Read the model definition and answer for the solid it produces. Units are mm, in the model's axes. Give positions to 0.01 mm unless a question says otherwise; leave off trailing zeros. Loops run counter-clockwise (first coordinate to the right, second up) from the corner with the lowest first, then second, coordinate; pieces in that order, holes last.
(1) Find section C-C, the plane x = -19. Write down the section's boundary in (y, z), then the cut area to 3 significant figures.
(2) Find section A-A, the plane y = 572. Write down the section's boundary in (x, z), then the cut area to 3 significant figures.
(3) Find section B-B, the plane z = -23. Write down the section's boundary in (x, y).
(4) Each of these flat-tipped pins is pushed along its axis until it touches: P1, Ø1, axis at y = 209, z = 25.5, coming from the +X side (3 decimals); P2, Ø5, axis at y = 8.5, z = 5.5, coming from the -X side; P3, Ø1, axis at x = 19, y = 293, coming from the +Z side; P4, Ø3, axis at y = -139.7, z = 0, coming from the +X side. Where does it stop, or does it pass through?
(5) Find section D-D, the plane y = -26. Write down the section's boundary in (x, z).
(6) Straight lines are drawn through the part: probe 1 along Y at (x, z) = (2.75, 0); probe 2 along Z at (x, y) = (4.5, -139.7); probe 3 along Y at (x, z) = (-16, 22). For each, find the intervals that lie inside material, in ascending order.
```python
from build123d import *

# Parameters (mm, degrees)
F0_R     = 32
F0_R_2   = 10
F1_DEPTH = 596.9
F2_DEPTH = 152.4
F3_R     = 10
F4_DEPTH = 152.4
F5_R     = 2.5
F5_R_2   = 2.5019
F6_DEPTH = 63.5


# Not quite as in the source:
# - a feature names something its author has since deleted; it is built from what else it names


with BuildPart() as f1:
    # F0 (on Front) → F1 (new body)
    with BuildSketch(Plane.XZ):
        Circle(F0_R)
        Circle(F0_R_2, mode=Mode.SUBTRACT)
        Circle(F0_R_2)
    extrude(amount=-F1_DEPTH)

    # F0 (on Front) → F2 (join)
    with BuildSketch(Plane.XZ):
        Circle(F0_R_2)
    extrude(amount=F2_DEPTH)

    # F3 (on face) → F4 (join)
    with BuildSketch(Plane(origin=(0, 596.9, 0), x_dir=(-1, 0, 0), z_dir=(0, 1, 0))):
        Circle(F3_R)
    extrude(amount=F4_DEPTH)

    # F5 (on Right) → F6 (cut, symmetric)
    with BuildSketch(Plane.YZ):
        with Locations((-139.7, 0)):
            Circle(F5_R)
        with Locations((737.87, 0)):
            Circle(F5_R_2)
    extrude(amount=F6_DEPTH, both=True, mode=Mode.SUBTRACT)


solid = f1.part
```
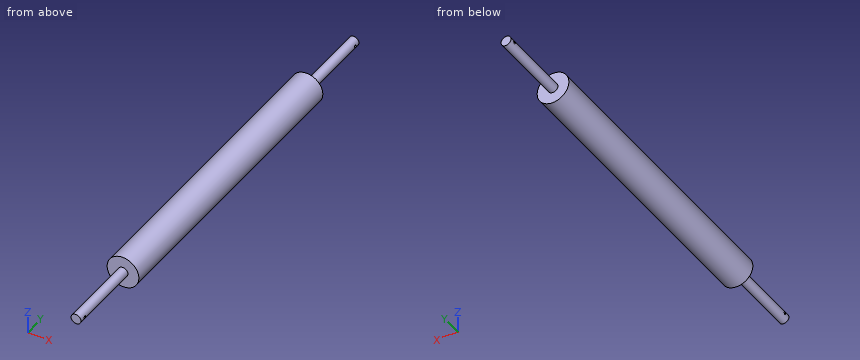
Entries:
1. outline: (0, -25.75) - (596.9, -25.75) - (596.9, 25.75) - (0, 25.75) - close
1. area: 30,700 mm2
2. outline: circle Ø64 at (0, 0)
2. area: 3,220 mm2
3. outline: (-22.25, 0) - (22.25, 0) - (22.25, 596.9) - (-22.25, 596.9) - close
4. P1: stops at x = 19.975
4. P2: stops at x = -31.86
4. P3: stops at z = 26.11
4. P4: passes through
5. outline: circle Ø20 at (0, 0)
6. probe 1: y = -152.4 to -142.2, -137.2 to 735.37, 740.37 to 749.3
6. probe 2: z = -8.93 to -2.5, 2.5 to 8.93
6. probe 3: y = 0 to 596.9
